Model file for the job. Use its own axes, mm. Round coordinates to 2 decimals unless told otherwise and drop trailing zeros. Write each loop counter-clockwise with the first axis right and the second up, starting at its lowest first coordinate (ties: lowest second). Pieces come first, ordered by that corner, then holes. Notation, with made-up numbers: (46.5, 83.25) - (77.5, 83.25) arc R22 cw to (77.5, 113.25) - close; hole circle Ø11 at (-32.75, -36). An arc over 180 degrees is marked (long way). One line per item, written item: value.
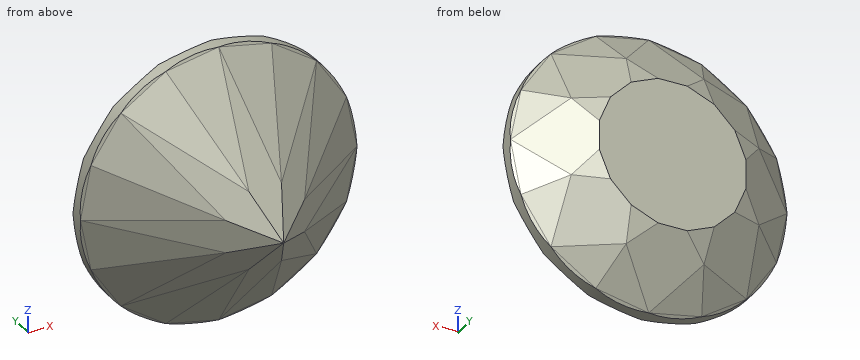
from build123d import *

# Parameters (mm, degrees)
ESQUISSE1_R                  = 5
BOSS_EXTRU_4_DEPTH           = 0.5
BOSS_EXTRU_5_DEPTH           = 4.32
BOSS_EXTRU_6_DEPTH           = 1.6
ENL_V_MAT_EXTRU_1_DEPTH      = 6
R_P_TITION_CIRCULAIRE1_COUNT = 8
ENL_V_MAT_EXTRU_4_DEPTH      = 7.935199227
R_P_TITION_CIRCULAIRE2_COUNT = 16
ENL_V_MAT_EXTRU_5_DEPTH      = 7.532814824
R_P_TITION_CIRCULAIRE3_COUNT = 8


with BuildPart() as part:
    # Esquisse1 → Boss.-Extru.4 (new body)
    with BuildSketch(Plane(origin=(0, 0, 0), x_dir=(1, 0, 0), z_dir=(0, 1, 0))):
        with Locations(Location((0, 0, 0), (0, 0, 270))):  # turned: the seam where the file's is
            Circle(ESQUISSE1_R)
    extrude(amount=BOSS_EXTRU_4_DEPTH)

    # Esquisse1_4 → Boss.-Extru.5 (add)
    with BuildSketch(Plane(origin=(0, 0, 0), x_dir=(1, 0, 0), z_dir=(0, 1, 0))):
        Polygon((2.832272487, -4.238795325), (4.238795325, -2.832272487), (5, -0.994561837), (5, 0.994561837), (4.238795325, 2.832272487), (2.832272487, 4.238795325), (0.994561837, 5), (-0.994561837, 5), (-2.832272487, 4.238795325), (-4.238795325, 2.832272487), (-5, 0.994561837), (-5, -0.994561837), (-4.238795325, -2.832272487), (-2.832272487, -4.238795325), (-0.994561837, -5), (0.994561837, -5), align=None)
    extrude(amount=-BOSS_EXTRU_5_DEPTH)

    # Esquisse11 → Boss.-Extru.6 (add)
    with BuildSketch(Plane(origin=(0, 0.5, 0), x_dir=(1, 0, 0), z_dir=(0, 1, 0))):
        Polygon((-0.994561837, 5), (-2.832272487, 4.238795325), (-4.238795325, 2.832272487), (-5, 0.994561837), (-5, -0.994561837), (-4.238795325, -2.832272487), (-2.832272487, -4.238795325), (-0.994561837, -5), (0.994561837, -5), (2.832272487, -4.238795325), (4.238795325, -2.832272487), (5, -0.994561837), (5, 0.994561837), (4.238795325, 2.832272487), (2.832272487, 4.238795325), (0.994561837, 5), align=None)
    extrude(amount=BOSS_EXTRU_6_DEPTH)

    # Esquisse7 → Enl_v. mat.-Extru.1 (cut, symmetric)
    with BuildSketch(Plane.XY):
        Polygon((-7, 0), (-7, -4.32), (-0.030408481, -4.32), (-5, 0), (-5, 0.5), (-2.65, 2.1), (-7, 2.1), align=None)
    enl_v_mat_extru_1 = extrude(amount=ENL_V_MAT_EXTRU_1_DEPTH, both=True, mode=Mode.SUBTRACT)

    # R_p_tition circulaire1: Enl_v. mat.-Extru.1 ×8 about axis
    r_p_tition_circulaire1_axis = Axis((0, 0, 0), (0, 1, 0))
    for i in range(1, R_P_TITION_CIRCULAIRE1_COUNT):
        add(enl_v_mat_extru_1.rotate(r_p_tition_circulaire1_axis, i * 360 / R_P_TITION_CIRCULAIRE1_COUNT), mode=Mode.SUBTRACT)

    # Esquisse10 → Enl_v. mat.-Extru.4 (cut, symmetric)
    with BuildSketch(Plane(origin=(0, 0, 0), x_dir=(-0.831469612, 0, -0.555570233), z_dir=(0.555570233, 0, -0.831469612))):
        Polygon((5.903926402, 0), (5.903926402, -4.86712571), (-0.407609261, -4.86712571), (4.903926402, 0), (5.221818983, 0.232853051), (4.903926402, 0.5), (3, 2.1), (5.903926402, 2.1), align=None)
    enl_v_mat_extru_4 = extrude(amount=ENL_V_MAT_EXTRU_4_DEPTH, both=True, mode=Mode.SUBTRACT)

    # R_p_tition circulaire2: Enl_v. mat.-Extru.4 ×16 about axis
    r_p_tition_circulaire2_axis = Axis((0, 0, 0), (0, 1, 0))
    for i in range(1, R_P_TITION_CIRCULAIRE2_COUNT):
        add(enl_v_mat_extru_4.rotate(r_p_tition_circulaire2_axis, i * 360 / R_P_TITION_CIRCULAIRE2_COUNT), mode=Mode.SUBTRACT)

    # Esquisse13 → Enl_v. mat.-Extru.5 (cut, symmetric)
    with BuildSketch(Plane(origin=(0, 0, 0), x_dir=(-0.923879533, 0, -0.382683432), z_dir=(0.382683432, 0, -0.923879533))):
        Polygon((3.672450086, 1.594194745), (2.65, 2.1), (3.922671549, 2.1), align=None)
        Polygon((-3.922671549, 2.1), (-3.672450086, 1.594194745), (-2.65, 2.1), align=None)
    enl_v_mat_extru_5 = extrude(amount=ENL_V_MAT_EXTRU_5_DEPTH, both=True, mode=Mode.SUBTRACT)

    # R_p_tition circulaire3: Enl_v. mat.-Extru.5 ×8 about axis
    r_p_tition_circulaire3_axis = Axis((0, 0, 0), (0, 1, 0))
    for i in range(1, R_P_TITION_CIRCULAIRE3_COUNT):
        add(enl_v_mat_extru_5.rotate(r_p_tition_circulaire3_axis, i * 360 / R_P_TITION_CIRCULAIRE3_COUNT), mode=Mode.SUBTRACT)


solid = part.part
1. Band-saw the part on D-D on x = -3.75. Write the cut outline in (y, z), plus the area to 3 significant figures.
Report:
outline: (-1.09, -0.21) - (-0.85, -1.55) - (0, -3.21) - (0.04, -3.31) - (0.46, -3.31) - (1.28, -1.55) - (1.35, -1.09) - (1.35, 1.09) - (1.28, 1.55) - (0.46, 3.31) - (0.04, 3.31) - (0, 3.21) - (-0.85, 1.55) - (-1.09, 0.21) - close
area: 11.7 mm²
2. Wall check: probe 1 along Y at (x, z) = (-2.5, 0); probe 2 along Y at (x, z) = (2.75, 3.5); probe 3 along Z at (x, y) = (-0.25, -2.75). Give the ranges that are in metal, low to high. Write a range as [from, to].
Report:
probe 1: [-2.17, 2.1]
probe 2: [-0.43, 0.89]
probe 3: [-1.84, 1.84]
3. Drop flat-ended pins along their axis: pin 1 (3 mm diameter, centred on x = -3.5, z = -2, fed in from -Y); pin 2 (1.5 mm diameter, centred on x = 3, y = -2, fed in from -Z). Give the stop position or say it passes through.
Report:
pin 1: y = -2.18
pin 2: z = -2.25
4. Band-saw the part on A-A on x = 0.25. Write the cut outline in (y, z), plus the area to 3 significant figures.
Report:
outline: (-4.13, -0.1) - (-3.82, -0.6) - (-1.32, -3.48) - (0, -4.95) - (0.03, -4.99) - (0.46, -4.99) - (0.69, -4.71) - (2.1, -2.65) - (2.1, 2.65) - (0.69, 4.71) - (0.46, 4.99) - (0.03, 4.99) - (0, 4.95) - (-1.32, 3.48) - (-3.82, 0.6) - (-4.13, 0.1) - close
area: 38.8 mm²
5. Band-saw the part on C-C on z = -0.25. Write the cut outline in (x, y).
Report:
outline: (-4.99, 0.03) - (-4.95, 0) - (-3.48, -1.32) - (-0.6, -3.82) - (-0.1, -4.13) - (0.1, -4.13) - (0.6, -3.82) - (3.48, -1.32) - (4.95, 0) - (4.99, 0.03) - (4.99, 0.46) - (4.71, 0.69) - (2.65, 2.1) - (-2.65, 2.1) - (-4.71, 0.69) - (-4.99, 0.46) - close
6. Band-saw the part on B-B on y = -1.75. Write the cut outline in (x, z), plus the area to 3 significant figures.
Report:
outline: (-2.99, -0.33) - (-2.82, -1.17) - (-2.35, -1.88) - (-1.88, -2.35) - (-1.17, -2.82) - (-0.33, -2.99) - (0.33, -2.99) - (1.17, -2.82) - (1.88, -2.35) - (2.35, -1.88) - (2.82, -1.17) - (2.99, -0.33) - (2.99, 0.33) - (2.82, 1.17) - (2.35, 1.88) - (1.88, 2.35) - (1.17, 2.82) - (0.33, 2.99) - (-0.33, 2.99) - (-1.17, 2.82) - (-1.88, 2.35) - (-2.35, 1.88) - (-2.82, 1.17) - (-2.99, 0.33) - close
area: 28.4 mm²
